Geometry check sheet. Reference: the model listing, model coordinates, mm. Face numbers are marked on the shaded views. A direction names the side the tool comes from. Round coordinates to 2 decimals unless told otherwise and drop trailing zeros. Write each loop counter-clockwise with the first axis right and the second up, starting at its lowest first coordinate (ties: lowest second). Pieces come first, ordered by that corner, then holes. Notation, with made-up numbers: M 50,78 L 78,78 A37 cw 78,116 Z; hole C -25.75,-13.5 d10. An arc over 180 degrees is marked long. Answer in a Markdown table with one row per item. Add a question column.
from build123d import *

# Parameters (mm, degrees)
ESQUISSE3_R                  = 1.5
ENL_V_MAT_EXTRU_1_DEPTH      = 5
R_P_TITION_CIRCULAIRE1_COUNT = 3
ESQUISSE4_R                  = 8
BOSS_EXTRU_1_DEPTH           = 2
BOSS_EXTRU_2_DEPTH           = 14
ENL_V_START                  = -8
ENL_V_MAT_EXTRU_2_DEPTH      = 16
ESQUISSE7_R                  = 5.5
BOSS_EXTRU_4_DEPTH           = 11
ESQUISSE8_R                  = 2.5
BOSS_EXTRU_5_DEPTH           = 10


# Read off the part's stored shape, not the designer's step: Enlèv. mat.-Extru.2
with BuildPart() as part:
    # Esquisse1 → Révolution1 (revolve)
    with BuildSketch(Plane.XY, mode=Mode.PRIVATE) as r_volution1_sk:
        Polygon((-13.555229236, 0), (-13.555229236, 15), (-39.555229236, 15), (-39.555229236, 2.5), (-54.555229236, 2.5), (-54.555229236, 0), align=None)
    revolve(r_volution1_sk.sketch.rotate(Axis((-72.521066027, 0, 0), (1, 0, 0)), 90), axis=Axis((-72.521066027, 0, 0), (1, 0, 0)))

    # Esquisse3 → Enlèv. mat.-Extru.1 (cut)
    with BuildSketch(Plane.ZY.offset(39.555229236)):
        with Locations((0, -12)):
            Circle(ESQUISSE3_R)
    enl_v_mat_extru_1 = extrude(amount=-ENL_V_MAT_EXTRU_1_DEPTH, mode=Mode.SUBTRACT)

    # Répétition circulaire1: Enlèv. mat.-Extru.1 ×3 about axis
    r_p_tition_circulaire1_axis = Axis((0, 0, 0), (1, 0, 0))
    for i in range(1, R_P_TITION_CIRCULAIRE1_COUNT):
        add(enl_v_mat_extru_1.rotate(r_p_tition_circulaire1_axis, i * 360 / R_P_TITION_CIRCULAIRE1_COUNT), mode=Mode.SUBTRACT)

    # Esquisse4 → Boss.-Extru.1 (add)
    with BuildSketch(Plane.ZY.offset(39.555229236)):
        with Locations(Location((0, 0, 0), (0, 0, 180))):
            Circle(ESQUISSE4_R)
    extrude(amount=BOSS_EXTRU_1_DEPTH)

    # Esquisse3D1 → Boss.-Extru.2 (add)
    with BuildSketch(Plane(origin=(-13.555229236, 12.68857754, 8), x_dir=(0, 0, -1), z_dir=(1, 0, 0))):
        Polygon((0, 0), (2, 3.464101615), (14, 3.464101615), (16, 0), align=None)
    extrude(amount=-BOSS_EXTRU_2_DEPTH)

    # Enlèv. mat.-Extru.2 outline → Enlèv. mat.-Extru.2 (cut)
    with BuildSketch(Plane.XY.offset(ENL_V_START)):
        Polygon((-27.555229236, 16.152679156), (-27.555229236, 12.68857754), (-24.555229236, 16.152679156), align=None)
    extrude(amount=ENL_V_MAT_EXTRU_2_DEPTH, mode=Mode.SUBTRACT)

    # Esquisse7 → Boss.-Extru.4 (add)
    with BuildSketch(Plane(origin=(0, 16.152679156, 0), x_dir=(1, 0, 0), z_dir=(0, 1, 0))):
        with Locations(Location((-19.055229236, 0, 0), (0, 0, 180))):
            Circle(ESQUISSE7_R)
    extrude(amount=BOSS_EXTRU_4_DEPTH)

    # Esquisse8 → Boss.-Extru.5 (add)
    with BuildSketch(Plane(origin=(0, 27.152679156, 0), x_dir=(1, 0, 0), z_dir=(0, 1, 0))):
        with Locations(Location((-19.055229236, 0, 0), (0, 0, 270))):
            Circle(ESQUISSE8_R)
    extrude(amount=BOSS_EXTRU_5_DEPTH)


solid = part.part
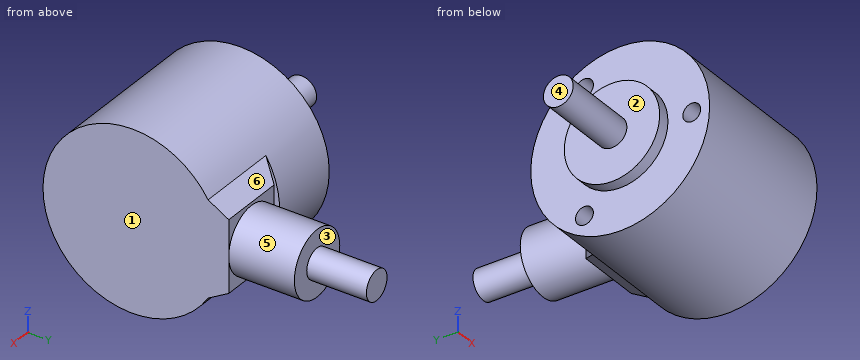
Item 1: Section check C-C, the plane x = -44.5. Record the boundary of the cut face in (y, z), and give its area (3 significant figures).
Item 2: Access from +Z, -Z, +X, -X, +Y, -Y to the whole of each face (thin tool, end or side, straight path). Record for the marked faces 1, 2 and 3.
Item 3: Gauge pin test, flat ends, axial feed: pin 1 Ø1.8 at (x, z) = (-19, 3.5) entering from +Y; pin 2 Ø10 at (x, z) = (-50, -1) entering from +Y; pin 3 Ø3.5 at (y, z) = (-12, 0) entering from -X. Record the tip position at first contact, or that the pin passes through.
Item 4: Section check B-B, the plane y = -12. Record the boundary of the cut face in (x, z).
Item 5: Mould release check, pull along Z, two halves, no side actions. Record for the marked faces 4, 5 and 6: +Z half, -Z half, draft (parallel to the pull), parting line (faces both ways), or undercut.
Item 6: Section check D-D, the plane y = 6. Record the boundary of the cut face in (x, z).
Item 7: Section check A-A, the plane y = 0. Record the boundary of the cut face in (x, z).
Item 8: Scan lines: probe 1 along Y at (x, z) = (-37.85, 0); probe 2 along X at (y, z) = (4.5, 9.75); probe 3 along X at (y, z) = (-1.5, 6). Record each from-to range of solid material in increasing order. Write a range as from..to.
Result sheet:
| question | item | result |
|---|---|---|
| 1 | outline | C 0,0 d5 |
| 1 | area | 19.6 mm^2 |
| 2 | face 1 | +Z, -Z, +X, +Y, -Y |
| 2 | face 2 | -X |
| 2 | face 3 | +Y |
| 3 | pin 1 | stops at y = 27.15 |
| 3 | pin 2 | stops at y = 2.5 |
| 3 | pin 3 | stops at x = -39.56 |
| 4 | outline | M -39.56,-9 L -13.56,-9 L -13.56,9 L -39.56,9 L -39.56,1.5 L -34.56,1.5 L -34.56,-1.5 L -39.56,-1.5 Z |
| 5 | face 4 | draft |
| 5 | face 5 | parting line |
| 5 | face 6 | +Z half |
| 6 | outline | M -41.56,-5.29 L -39.56,-5.29 L -39.56,-8.89 L -34.56,-8.89 L -34.56,-11.89 L -39.56,-11.89 L -39.56,-13.75 L -13.56,-13.75 L -13.56,13.75 L -39.56,13.75 L -39.56,11.89 L -34.56,11.89 L -34.56,8.89 L -39.56,8.89 L -39.56,5.29 L -41.56,5.29 Z |
| 7 | outline | M -54.56,-2.5 L -41.56,-2.5 L -41.56,-8 L -39.56,-8 L -39.56,-15 L -13.56,-15 L -13.56,15 L -39.56,15 L -39.56,8 L -41.56,8 L -41.56,2.5 L -54.56,2.5 Z |
| 8 | probe 1 | y = -15..-13.5, -10.5..15 |
| 8 | probe 2 | x = -39.56..-13.56 |
| 8 | probe 3 | x = -41.56..-13.56 |
